The drawing under review shows one solid part. Ordinate dimensions are in mm from its lowest x, y, z. Give positions to 0.01 mm unless a question says otherwise; leave off trailing zeros. Order: outer loops, then holes, each group sorted by start corner. A loop starts at its lowest first (then second) coordinate and runs counter-clockwise, first axis right, second up. Notation, with made-up numbers: (49.25, -33) - (53.25, -33) arc R29 cw to (53.25, 1) - close; hole circle Ø1 at (50.5, 68). An arc over 180 degrees is marked (long way). Use CSV: the item, a comma, the result in double quotes.
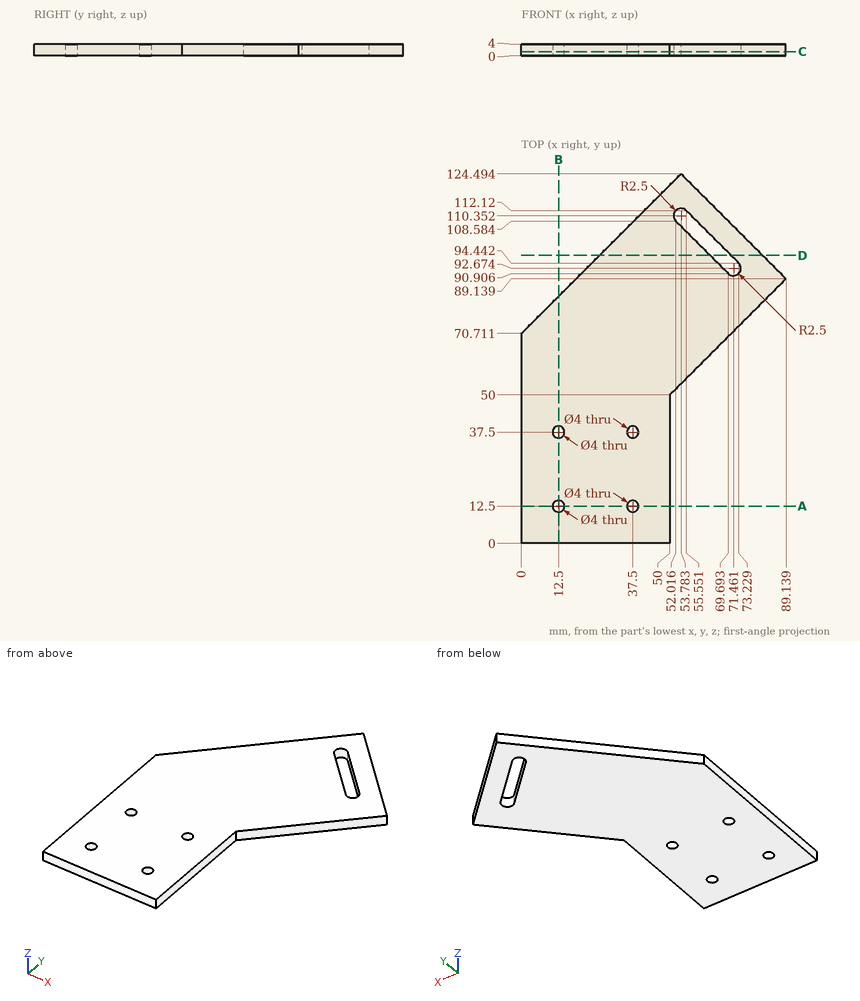
Item 1: Take a section at C-C, the plane z = 1.4. Give the boundary of the cut face in (x, y) (1 decimal), and give its area (3 significant figures).
Results list:
outline,"(0, 0) - (50, 0) - (50, 50) - (89.1, 89.1) - (53.8, 124.5) - (0, 70.7) - close; hole circle Ø4 at (12.5, 12.5); hole circle Ø4 at (12.5, 37.5); hole circle Ø4 at (37.5, 12.5); hole circle Ø4 at (37.5, 37.5); hole (52, 108.6) - (69.7, 90.9) arc R2.5 ccw to (73.2, 94.4) - (55.6, 112.1) arc R2.5 ccw to start"
area,"6,110 mm2"
Item 2: Wall thickness on L1, parallel to Y at x = 38, z = 2.75 (1 decimal); L2, parallel to Y at x = 12.5, z = 2.25; L3, parallel to X at y = 9, z = 3.55: over which ranges is each line inside the solid? List them lowest first.
Results list:
L1,"y = 0 to 10.6, 14.4 to 35.6, 39.4 to 108.7"
L2,"y = 0 to 10.5, 14.5 to 35.5, 39.5 to 83.21"
L3,"x = 0 to 50"
Item 3: Take a section at D-D, the plane y = 97. Give the boundary of the cut face in (x, z).
Results list:
outline,"(26.29, 0) - (63.6, 0) - (63.6, 4) - (26.29, 4) - close; (70.67, 0) - (81.28, 0) - (81.28, 4) - (70.67, 4) - close"
Item 4: Take a section at B-B, the plane x = 12.5. Give the boundary of the cut face in (y, z), and give its area (3 significant figures).
Results list:
outline,"(0, 0) - (10.5, 0) - (10.5, 4) - (0, 4) - close; (14.5, 0) - (35.5, 0) - (35.5, 4) - (14.5, 4) - close; (39.5, 0) - (83.21, 0) - (83.21, 4) - (39.5, 4) - close"
area,"301 mm2"
Item 5: Clearance check with flat-ended pins moving along their axes: pin 1 (3.5 mm diameter, centred on x = 37.5, y = 12.5, fed in from +Z); pin 2 (1.2 mm diameter, centred on y = 21, z = 1.5, fed in from +X); pin 3 (6.5 mm diameter, centred on x = 12.5, y = 12.5, fed in from +Z). State where each tip first meets the part, or that it passes through.
Results list:
pin 1,"passes through"
pin 2,"stops at x = 50"
pin 3,"stops at z = 4"
Item 6: Take a section at A-A, the plane y = 12.5. Give the boundary of the cut face in (x, z).
Results list:
outline,"(0, 0) - (10.5, 0) - (10.5, 4) - (0, 4) - close; (14.5, 0) - (35.5, 0) - (35.5, 4) - (14.5, 4) - close; (39.5, 0) - (50, 0) - (50, 4) - (39.5, 4) - close"
